Could you check a few things on this model? Use its own coordinates, in mm. A direction names the side the tool comes from. Coordinates: 2 decimals unless noted, no trailing zeros. Loops run counter-clockwise (first coordinate to the right, second up) from the corner with the lowest first, then second, coordinate; pieces in that order, holes last.
1) If I drill on line 1 along X through (y, z) = (4, 200); line 2 along X through (y, z) = (5.25, 160.5); line 3 along X through (y, z) = (2.75, 30), over which ranges is the centre line in solid material (lowest first)?
2) Imagine slicing it at B-B on z = 200. Please give me the cut outline in (x, y).
3) Imagine slicing it at C-C on z = 107. Please give me the cut outline in (x, y), plus the area to 3 significant figures.
4) Will these pins go through, and if not, where does the flat tip stop? P1, Ø6, axis at x = 113, z = 171, coming from the -Y side; P2, Ø3, axis at y = 3.5, z = 31.5, coming from the -X side; P3, Ø1.9, axis at y = 2, z = 129, coming from the +X side; P4, Ø1, axis at y = 4, z = 43.5, coming from the +X side.
5) Imagine slicing it at A-A on x = 80. Please give me the cut outline in (y, z).
6) Imagine slicing it at D-D on x = 186. Please give me the cut outline in (y, z).
7) Thinking about a two-plate mould opening in Z: for faces 1 (the face through (-89.54, 3.13, 196.48)), 2 (the face through (83, 6.35, 157)), 3 (the face through (214.23, 3.13, 64.09)), 4 (the face through (198.93, 3.22, 86.73)), which applies, released by +Z, released by -Z, zero draft, split by the parting line, or undercut?
8) For faces 5 (the face through (15.58, 3.22, 64)), 6 (the face through (-55.77, 3.13, 65.91)), which set-ups out of +Z, -Z, +X, -X, +Y, -Y let a thin tool reach every point of the face, with its end or its side?
```python
from build123d import *

# Parameters (mm, degrees)
BOSS_EXTRUDE1_DEPTH                 = 6.35
M5X0_8_TAPPED_HOLE1_D               = 4.2
F_7_1_7_1_DIAMETER_HOLE1_D          = 7.1
F_5_0MM_CLEARANCE_DOWEL_SLOT2_DEPTH = 6.35
CUT_EXTRUDE1_DEPTH                  = 10
SKETCH18_W                          = 110
SKETCH18_H                          = 40.64
CUT_EXTRUDE2_DEPTH                  = 10
FILLET1_R                           = 4
FILLET1_OF_MIRROR1_R                = 4


# Read off the part's stored shape, not the designer's step: Ø5.0mm Clearance Dowel Slot2
with BuildPart() as part:
    # Sketch1 → Boss-Extrude1 (new body)
    with BuildSketch(Plane(origin=(0, 0, 0), x_dir=(1, 0, 0), z_dir=(0, 1, 0))):
        Polygon((0, 0), (160, 0), (270, -130), (270, -220), (-110, -220), (-110, -130), align=None)
    extrude(amount=BOSS_EXTRUDE1_DEPTH)

    # M5x0.8 Tapped Hole1 (through all)
    with Locations(Plane(origin=(0, 6.35, 0), x_dir=(1, 0, 0), z_dir=(0, 1, 0))):
        with Locations((10, -10), (150, -10), (150, -30), (10, -30), (30, -50), (50, -50), (110, -50), (130, -50), (90, -10), (90, -30), (70, -10), (70, -30), (70, -210), (90, -210), (50, -190), (110, -190)):
            Hole(M5X0_8_TAPPED_HOLE1_D / 2)

    # Ø7.1 (7.1) Diameter Hole1 (through all)
    with Locations(Plane(origin=(0, 6.35, 0), x_dir=(1, 0, 0), z_dir=(0, 1, 0))):
        with Locations((250, -139.36), (250, -200), (-90, -200), (-90, -139.36)):
            Hole(F_7_1_7_1_DIAMETER_HOLE1_D / 2)

    # Ø5.0mm Clearance Dowel Slot2 outline → Ø5.0mm Clearance Dowel Slot2 (cut)
    with BuildSketch(Plane(origin=(0, 0, 0), x_dir=(1, 0, 0), z_dir=(0, 1, 0))):
        with BuildLine():
            Line((58.98, -90.31), (58.98, -75.41))
            ThreePointArc((58.98, -75.41), (56.43, -72.86), (53.88, -75.41))
            Line((53.88, -75.41), (53.88, -90.31))
            ThreePointArc((53.88, -90.31), (56.43, -92.86), (58.98, -90.31))
        make_face()
        with BuildLine():
            ThreePointArc((58.98, -122.55), (56.43, -120), (53.88, -122.55))
            Line((53.88, -122.55), (53.88, -137.45))
            ThreePointArc((53.88, -137.45), (56.43, -140), (58.98, -137.45))
            Line((58.98, -137.45), (58.98, -122.55))
        make_face()
        with BuildLine():
            Line((106.12, -90.31), (106.12, -75.41))
            ThreePointArc((106.12, -75.41), (103.57, -72.86), (101.02, -75.41))
            Line((101.02, -75.41), (101.02, -90.31))
            ThreePointArc((101.02, -90.31), (103.57, -92.86), (106.12, -90.31))
        make_face()
        with BuildLine():
            ThreePointArc((106.12, -122.55), (103.57, -120), (101.02, -122.55))
            Line((101.02, -122.55), (101.02, -137.45))
            ThreePointArc((101.02, -137.45), (103.57, -140), (106.12, -137.45))
            Line((106.12, -137.45), (106.12, -122.55))
        make_face()
    extrude(amount=F_5_0MM_CLEARANCE_DOWEL_SLOT2_DEPTH, mode=Mode.SUBTRACT)

    # Sketch17 → Cut-Extrude1 (cut)
    with BuildSketch(Plane(origin=(0, 6.35, 0), x_dir=(1, 0, 0), z_dir=(0, 1, 0))):
        with BuildLine():
            Line((100, -96.43), (100, -116.43))
            ThreePointArc((100, -116.43), (80, -136.43), (60, -116.43))
            Line((60, -116.43), (60, -96.43))
            ThreePointArc((60, -96.43), (80, -76.43), (100, -96.43))
        make_face()
    extrude(amount=-CUT_EXTRUDE1_DEPTH, mode=Mode.SUBTRACT)

    # Sketch18 → Cut-Extrude2 (cut)
    with BuildSketch(Plane(origin=(0, 6.35, 0), x_dir=(1, 0, 0), z_dir=(0, 1, 0))):
        Polygon((-75, -129.36), (-4.975810347, -46.6041395), (35, -80.429825178), (35, -129.36), align=None)
        with Locations((-20, -169.68)):
            Rectangle(SKETCH18_W, SKETCH18_H)
    cut_extrude2 = extrude(amount=-CUT_EXTRUDE2_DEPTH, mode=Mode.SUBTRACT)

    # Fillet1
    fillet1_edges = [part.edges().sort_by_distance(p)[0] for p in [
        (-75, 3.175, 190),
        (-75, 3.175, 149.36),
        (35, 3.175, 149.36),
        (35, 3.175, 190),
        (35, 3.175, 129.36),
        (-75, 3.175, 129.36),
        (-4.975810347, 3.175, 46.6041395),
        (35, 3.175, 80.429825178),
    ]]
    fillet(fillet1_edges, radius=FILLET1_R)

    # Mirror1: Cut-Extrude2 across plane
    add(cut_extrude2.mirror(Plane.ZY.offset(-80)), mode=Mode.SUBTRACT)

    # Fillet1 of Mirror1
    fillet1_of_mirror1_edges = [part.edges().sort_by_distance(p)[0] for p in [
        (235, 3.175, 190),
        (235, 3.175, 149.36),
        (125, 3.175, 149.36),
        (125, 3.175, 190),
        (125, 3.175, 129.36),
        (235, 3.175, 129.36),
        (164.975810347, 3.175, 46.6041395),
        (125, 3.175, 80.429825178),
    ]]
    fillet(fillet1_of_mirror1_edges, radius=FILLET1_OF_MIRROR1_R)


solid = part.part
```
Filled in:
1. line 1: x = -110 to -93.55, -86.45 to 246.45, 253.55 to 270
1. line 2: x = -110 to -75, 35 to 125, 235 to 270
1. line 3: x = -25.38 to 7.9, 12.1 to 67.9, 72.1 to 87.9, 92.1 to 147.9, 152.1 to 185.38
2. outline: (-110, 0) - (-93.55, 0) - (-93.55, 6.35) - (-110, 6.35) - close; (-86.45, 0) - (246.45, 0) - (246.45, 6.35) - (-86.45, 6.35) - close; (253.55, 0) - (270, 0) - (270, 6.35) - (253.55, 6.35) - close
3. outline: (-90.54, 0) - (-56.08, 0) - (-56.08, 6.35) - (-90.54, 6.35) - close; (35, 0) - (60, 0) - (60, 6.35) - (35, 6.35) - close; (100, 0) - (125, 0) - (125, 6.35) - (100, 6.35) - close; (216.08, 0) - (250.54, 0) - (250.54, 6.35) - (216.08, 6.35) - close
3. area: 755 mm2
4. P1: stops at y = 0
4. P2: stops at x = -27.92
4. P3: stops at x = 269.96
4. P4: stops at x = 197.23
5. outline: (0, 0) - (6.35, 0) - (6.35, 76.43) - (0, 76.43) - close; (0, 136.43) - (6.35, 136.43) - (6.35, 220) - (0, 220) - close
6. outline: (0, 30.73) - (6.35, 30.73) - (6.35, 71.45) - (0, 71.45) - close; (0, 129.36) - (6.35, 129.36) - (6.35, 149.36) - (0, 149.36) - close; (0, 190) - (6.35, 190) - (6.35, 220) - (0, 220) - close
7. face 1: undercut
7. face 2: zero draft
7. face 3: released by -Z
7. face 4: undercut
8. face 5: +Y, -Y
8. face 6: -Z, -X, +Y, -Y
